Autodesk Inventor part; units mm, degrees
ref_plane "YZ Plane" through (0, 0, 0) normal (1, 0, 0) x (0, 1, 0)
ref_plane "XZ Plane" through (0, 0, 0) normal (0, 1, 0) x (-1, 0, 0)
ref_plane "XY Plane" through (0, 0, 0) normal (0, 0, 1) x (1, 0, 0)
sketch "Sketch1" plane through (0, 0, 0) normal (0, 1, 0) x (-1, 0, 0)
  circle A0 centre (0, 0) radius 12.5
  circle A1 centre (0, 0) radius 8
  dimension "d0" = 25
  dimension "d1" = 16
extrude "Extrusion1" add sketch "Sketch1" along normal blind 51
sketch "Sketch2" plane through (0, 51, 0) normal (0, 1, 0) x (1, 0, 0)
  circle A0 centre (0, 0) radius 12.25
  circle A1 centre (0, 0) radius 12.5
  dimension "d4" = 24.5
extrude "Extrusion2" cut sketch "Sketch2" against normal blind 0.5
sketch "Sketch3" plane through (0, 0, 0) normal (0, -1, 0) x (1, 0, 0)
  circle A0 centre (0, 0) radius 12.25
  circle A1 centre (0, 0) radius 12.5
  dimension "d7" = 24.5
extrude "Extrusion3" cut sketch "Sketch3" against normal blind 0.5
properties part number "P-025.40H Piezo Ring Actuators" material "Porcelain, Ivory"
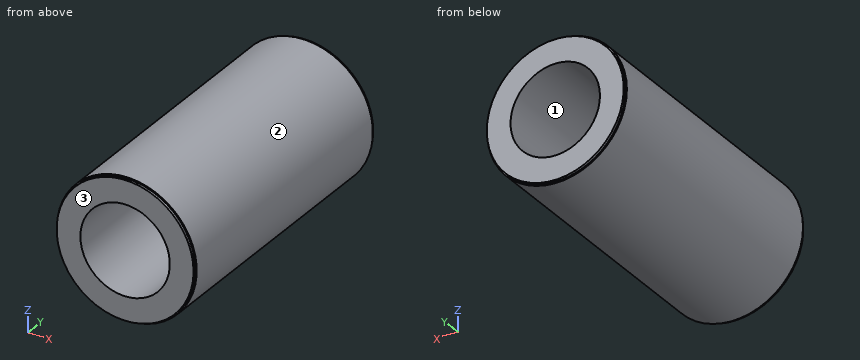
Check sheet for the modelled part. Datum: model origin and axes. Units: mm. Face numbers are marked on the shaded views. Give positions to 0.01 mm unless a question says otherwise; leave off trailing zeros. Write each loop counter-clockwise with the first axis right and the second up, starting at its lowest first coordinate (ties: lowest second). Pieces come first, ordered by that corner, then holes. Notation, with made-up numbers: M -38,35.5 L -3,35.5 A27 ccw -3,51.5 Z; hole C -19.75,-32.75 d9. An arc over 180 degrees is marked long. Use one line per item in the form item = value.
(1) Depth check by flat-ended pin: P1, Ø3, axis at x = 7, y = 34, coming from the +Z side (3 decimals); P2, Ø2, axis at y = 44.5, z = -6.5, coming from the +X side (3 decimals); P3, Ø1, axis at y = 7.5, z = -5, coming from the +X side. Enter the tip coordinate at first touch or a pass-through.
Answer block:
P1 = 11.225
P2 = 11.225
P3 = 11.66
(2) Section check C-C on y = 5.5. Record the boundary of the cut face in (x, z).
Answer block:
outline = C 0,0 d25; hole C 0,0 d16
(3) Material ranges on line 1 along Z through (x, y) = (0, 38.5); line 2 along X through (y, z) = (11.5, 6.75); line 3 along Z through (x, y) = (-3.5, 5.5), recorded low to high.
Answer block:
line_1 = -12.5 to -8, 8 to 12.5
line_2 = -10.52 to -4.29, 4.29 to 10.52
line_3 = -12 to -7.19, 7.19 to 12
(4) Section check B-B on z = 0. Record the boundary of the cut face in (x, y), plus the area to 4 significant figures.
Answer block:
outline = M -12.5,0.5 L -12.25,0.5 L -12.25,0 L -8,0 L -8,51 L -12.25,51 L -12.25,50.5 L -12.5,50.5 Z; M 8,0 L 12.25,0 L 12.25,0.5 L 12.5,0.5 L 12.5,50.5 L 12.25,50.5 L 12.25,51 L 8,51 Z
area = 458.5 mm2
(5) Draft check along Z on the marked faces 1, 2 and 3. Enter one of: pulls with the +Z half, pulls with the -Z half, needs draft (parallel to the pull), parting line crosses it, or undercut.
Answer block:
face_1 = undercut
face_2 = parting line crosses it
face_3 = needs draft
(6) Section check D-D on x = 10.5. Record the boundary of the cut face in (y, z), plus the area to 3 significant figures.
Answer block:
outline = M 0,-6.31 L 0.5,-6.31 L 0.5,-6.78 L 50.5,-6.78 L 50.5,-6.31 L 51,-6.31 L 51,6.31 L 50.5,6.31 L 50.5,6.78 L 0.5,6.78 L 0.5,6.31 L 0,6.31 Z
area = 691 mm2
(7) Section check A-A on x = 0. Record the boundary of the cut face in (y, z).
Answer block:
outline = M 0,-12.25 L 0.5,-12.25 L 0.5,-12.5 L 50.5,-12.5 L 50.5,-12.25 L 51,-12.25 L 51,-8 L 0,-8 Z; M 0,8 L 51,8 L 51,12.25 L 50.5,12.25 L 50.5,12.5 L 0.5,12.5 L 0.5,12.25 L 0,12.25 Z
